For this review, take the finished solid that the model builds, in its own axes (mm). A direction names the side the tool comes from. Give positions to 0.01 mm unless a question says otherwise; leave off trailing zeros. Order: outer loops, then holes, each group sorted by start corner. A loop starts at its lowest first (then second) coordinate and runs counter-clockwise, first axis right, second up. Notation, with made-up numbers: M 13.5,-7.75 L 42.5,-7.75 A28 ccw 42.5,19.25 Z; hole C 42,-9.5 d4. An arc over 180 degrees is marked long. Answer as CSV lines item,"result". Start each with the question number.
1. We need section D-D, the plane y = -7.25. Give the boundary of the cut face in (x, z), and give its area (3 significant figures).
2. We need section B-B, the plane z = 0. Give the boundary of the cut face in (x, y).
3. We need section C-C, the plane x = -2.54. Give the boundary of the cut face in (y, z).
4. Mouldability with a two-part tool opening along Z and no side actions: class faces 1 (the flat face through (0, -7, 5.5)), 2 (the flat face through (-1.3, -11.85, -1.3)), 3 (the flat face through (0, -7, 4.5)) as pulls with the +Z half, pulls with the -Z half, needs draft (parallel to the pull), parting line crosses it, or undercut.
5. For line 1 along Y through (x, z) = (-5.25, -0.25); line 2 along Y through (x, z) = (-4.5, -2.5); line 3 along Z through (x, y) = (3.75, -7.25), list the stretches that pass through material, from the lowest coordinate up.
6. Machinability: for faces 4 (the flat face through (-5.1, 1, 0)), 5 (the flat face through (2, -7, 5)), 6 (the flat face through (0, -7, -5.5)), which of the approach directions +Z, -Z, +X, -X, +Y, -Y give a long, thin tool a straight path to every point of the face, cutting with its end or side? Answer none if there is none.
7. We need section A-A, the plane y = -9.5. Give the boundary of the cut face in (x, z), and give its area (3 significant figures).
8. Clearance check with flat-ended pins moving along their axes: P1, Ø0.8, axis at x = -0.5, z = -5, coming from the -Y side; P2, Ø1.8, axis at x = -0.5, y = 1.5, coming from the +Z side; P3, Ø0.5, axis at y = -7.5, z = -5, coming from the +X side. State where each tip first meets the part, or that it passes through.
from build123d import *

# Parameters (mm, degrees)
SKETCH1_W           = 12.4
SKETCH1_H           = 12.4
BOSS_EXTRUDE1_DEPTH = 6.4
SKETCH2_W           = 10.2
SKETCH2_H           = 10.2
BOSS_EXTRUDE2_DEPTH = 2.3
SKETCH3_R           = 0.5
BOSS_EXTRUDE3_DEPTH = 5.45
SKETCH4_W           = 4
SKETCH4_H           = 1
BOSS_EXTRUDE4_DEPTH = 1.3


with BuildPart() as part:
    # Sketch1 → Boss-Extrude1 (new body)
    with BuildSketch(Plane(origin=(0, 0, 0), x_dir=(1, 0, 0), z_dir=(0, 1, 0))):
        Rectangle(SKETCH1_W, SKETCH1_H)
    extrude(amount=-BOSS_EXTRUDE1_DEPTH)

    # Sketch2 → Boss-Extrude2 (add)
    with BuildSketch(Plane(origin=(0, 0, 0), x_dir=(1, 0, 0), z_dir=(0, 1, 0))):
        Rectangle(SKETCH2_W, SKETCH2_H)
    extrude(amount=BOSS_EXTRUDE2_DEPTH)

    # Sketch3 → Boss-Extrude3 (add)
    with BuildSketch(Plane.XZ.offset(6.4)):
        with Locations(Location((-2.54, 1.27, 0), (0, 0, 270))):
            Circle(SKETCH3_R)
        Polygon((4.304974747, 4.022132034), (4.022132034, 4.304974747), (3.668578644, 3.951421356), (3.951421356, 3.668578644), align=None)
        Polygon((3.951421356, 3.668578644), (3.668578644, 3.951421356), (3.315025253, 3.597867966), (3.597867966, 3.315025253), align=None)
        with Locations(Location((3.81, -3.81, 0), (0, 0, 270))):
            Circle(SKETCH3_R)
        Polygon((-0.775025253, -1.482132034), (-1.128578644, -1.128578644), (-1.411421356, -1.411421356), (-1.057867966, -1.764974747), align=None)
        Polygon((-1.128578644, -1.128578644), (-1.482132034, -0.775025253), (-1.764974747, -1.057867966), (-1.411421356, -1.411421356), align=None)
    extrude(amount=BOSS_EXTRUDE3_DEPTH)

    # Sketch4 → Boss-Extrude4 (add)
    with BuildSketch(Plane.XZ.offset(6.4)):
        with Locations((0, -5)):
            Rectangle(SKETCH4_W, SKETCH4_H)
        with Locations((0, 5)):
            Rectangle(SKETCH4_W, SKETCH4_H)
    extrude(amount=BOSS_EXTRUDE4_DEPTH)


solid = part.part
Result set:
1,outline,"C -2.54,1.27 d1; M -2,-5.5 L 2,-5.5 L 2,-4.5 L -2,-4.5 Z; M -2,4.5 L 2,4.5 L 2,5.5 L -2,5.5 Z; M -1.76,-1.06 L -1.06,-1.76 L -0.78,-1.48 L -1.48,-0.78 Z; C 3.81,-3.81 d1; M 3.32,3.6 L 3.6,3.32 L 4.3,4.02 L 4.02,4.3 Z"
1,area,"10.4 mm2"
2,outline,"M -6.2,-6.4 L 6.2,-6.4 L 6.2,0 L 5.1,0 L 5.1,2.3 L -5.1,2.3 L -5.1,0 L -6.2,0 Z"
3,outline,"M -11.85,0.77 L -6.4,0.77 L -6.4,-6.2 L 0,-6.2 L 0,-5.1 L 2.3,-5.1 L 2.3,5.1 L 0,5.1 L 0,6.2 L -6.4,6.2 L -6.4,1.77 L -11.85,1.77 Z"
4,face 1,"pulls with the +Z half"
4,face 2,"needs draft"
4,face 3,"undercut"
5,line 1,"-6.4 to 0"
5,line 2,"-6.4 to 2.3"
5,line 3,"-4.31 to -3.31, 3.47 to 4.03"
6,face 4,"+Z, -Z, -X, +Y"
6,face 5,"+Z, -Z, +X, -Y"
6,face 6,"-Z, +X, -X, -Y"
7,outline,"C -2.54,1.27 d1; M -1.76,-1.06 L -1.06,-1.76 L -0.78,-1.48 L -1.48,-0.78 Z; C 3.81,-3.81 d1; M 3.32,3.6 L 3.6,3.32 L 4.3,4.02 L 4.02,4.3 Z"
7,area,"2.37 mm2"
8,P1,"y = -7.7"
8,P2,"z = 5.1"
8,P3,"x = 2"
